Check sheet for the modelled part. Datum: model origin and axes. Units: mm. A direction names the side the tool comes from. Coordinates: 2 decimals unless noted, no trailing zeros. Order: outer loops, then holes, each group sorted by start corner. A loop starts at its lowest first (then second) coordinate and runs counter-clockwise, first axis right, second up. Notation, with made-up numbers: M -17,20.5 L -12,20.5 A21 cw -12,50.5 Z; hole C 28.5,-17 d3. An arc over 180 degrees is marked long. Answer in a Markdown table with one row per item. Add a question column.
from build123d import *

# Parameters (mm, degrees)
BOSS_EXTRUDE1_DEPTH = 4
FILLET1_R           = 5
FILLET2_R           = 5
SKETCH6_R           = 1.5
CUT_EXTRUDE1_DEPTH  = 32.558605799


with BuildPart() as part:
    # Sketch2 → Boss-Extrude1 (new body)
    with BuildSketch(Plane(origin=(0, 0, 0), x_dir=(1, 0, 0), z_dir=(0, 1, 0))):
        Polygon((0, 0), (18.84, 0), (18.84, 25), (16.84, 25), (16.84, 18), (0, 16), align=None)
    extrude(amount=BOSS_EXTRUDE1_DEPTH)

    # Fillet1
    # the kernel refuses this fillet: 5 mm, written as the material it takes off along each edge
    with BuildSketch(Plane(origin=(-12.247448714, 4, 0), x_dir=(0, -1.0, -1.5634160632766466e-12), z_dir=(1, 0, 0))) as fillet1_piece_1:
        with BuildLine():
            CenterArc((5, 4.898979486), FILLET1_R, 180, 78.463040967)
            Line((0, 4.898979486), (-0.1, 4.898979486))
            Line((-0.1, 4.898979486), (-0.1, 0))
            Line((-0.1, 0), (0, -0.1))
            ThreePointArc((0, -0.1), (2, -0.1), (3.98, -0.09797959))
            Line((3.98, -0.09797959), (4, 0))
        make_face()
    extrude(amount=43.334897428, mode=Mode.SUBTRACT)

    # Fillet2
    fillet2_edges = [part.edges().sort_by_distance(p)[0] for p in [
        (16.84, 2, -18),
    ]]
    fillet(fillet2_edges, radius=FILLET2_R)

    # Sketch6 → Cut-Extrude1 (cut, through all)
    with BuildSketch(Plane(origin=(18.84, 0, 0), x_dir=(0, 0, -1), z_dir=(1, 0, 0))):
        with Locations((23, 2)):
            Circle(SKETCH6_R)
        with BuildLine():
            Line((25, 4), (23, 4))
            ThreePointArc((23, 4), (24.414213562, 3.414213562), (25, 2))
            Line((25, 2), (25, 4))
        make_face()
        with BuildLine():
            Line((25, 0), (25, 2))
            ThreePointArc((25, 2), (24.414213562, 0.585786438), (23, 0))
            Line((23, 0), (25, 0))
        make_face()
    extrude(amount=-CUT_EXTRUDE1_DEPTH, mode=Mode.SUBTRACT)


solid = part.part
1. Section check C-C on x = 9.5. Enter the section's corners in (y, z), then the cut area to 3 significant figures.
2. Section check B-B on x = 13.25. Enter the section's corners in (y, z).
3. Set-up check for faces 1 (the flat face through (0, 2, -8)), 2 (the flat face through (16.84, 2, -24.7)): record each of +Z, -Z, +X, -X, +Y, -Y from which the full face is reachable in a straight line by a thin tool's end or side.
4. Scan lines: line 1 (Y direction, x = 18.45, z = -23); line 2 (X direction, y = 0.3, z = -22.25); line 3 (Z direction, x = 17.35, y = 2). Record each from-to range of solid material in increasing order.
5. Section check A-A on y = 1.45. Enter the section's corners in (x, z), then the cut area to 3 significant figures.
6. Release check for a two-part mould opening along Y. For faces 3 (the cylindrical face through (17.81, 2.07, -21.5)), 4 (the flat face through (6.3, 1.97, -16.75)), 5 (the cylindrical face through (9.29, 2.9, -1.77)) record: released by +Y, released by -Y, zero draft, split by the parting line, or undercut.
7. Go/stop test with flat-tipped pins: pin 1 Ø8 at (x, z) = (10, -21) entering from +Y; pin 2 Ø0.8 at (y, z) = (2, -24.5) entering from -X. Record where each tip stops, or that it passes through.
Result sheet:
| question | item | result |
|---|---|---|
| 1 | outline | M 0,-17.13 L 4,-17.13 L 4,-4.9 A5 ccw 0,0 Z |
| 1 | area | 63.6 mm^2 |
| 2 | outline | M 0,-17.64 L 4,-17.64 L 4,-4.9 A5 ccw 0,0 Z |
| 3 | face 1 | +Z, -Z, -X, +Y, -Y |
| 3 | face 2 | -Z, -X, +Y, -Y |
| 4 | line 1 | 0 to 0.5, 3.5 to 4 |
| 4 | line 2 | 16.84 to 18.84 |
| 4 | line 3 | -25 to -24.5, -21.5 to -0.9 |
| 5 | outline | M 0,-16 L 12.43,-17.48 A5 cw 16.77,-21.6 L 18.84,-21.6 L 18.84,-0.54 L 0,-0.54 Z; M 16.84,-24.92 L 18.84,-24.92 L 18.84,-24.4 L 16.84,-24.4 Z |
| 5 | area | 324 mm^2 |
| 6 | face 3 | undercut |
| 6 | face 4 | zero draft |
| 6 | face 5 | released by +Y |
| 7 | pin 1 | y = 4 |
| 7 | pin 2 | x = 16.84 |
